Geometry: final body of the model. Coordinates: model frame, mm. A direction names the side the tool comes from. Give positions to 0.01 mm unless a question says otherwise; leave off trailing zeros. Order: outer loops, then holes, each group sorted by start corner. A loop starts at its lowest first (then second) coordinate and runs counter-clockwise, first axis right, second up. Notation, with made-up numbers: M 51,37 L 56,37 A19 ccw 56,60 Z; hole C 66.5,-2 d10. An arc over 180 degrees is marked long. Write item = value, one per line. Start each with the question number.
from build123d import *

# Parameters (mm, degrees)
SKETCH1_R                                     = 19.05
BOSS_EXTRUDE1_DEPTH                           = 2.54
CSK_FOR_4_FLAT_HEAD_MACHINE_SCREW1_AT_2_COUNT = 2
CSK_FOR_4_FLAT_HEAD_MACHINE_SCREW1_AT_2_PITCH = 26.396454307
CSK_FOR_4_FLAT_HEAD_MACHINE_SCREW1_AT_3_COUNT = 2
CSK_FOR_4_FLAT_HEAD_MACHINE_SCREW1_AT_3_PITCH = 26.396454307
F_57_0_043_DIAMETER_HOLE1_D                   = 1.0922
SKETCH9_R                                     = 2.921
BOSS_EXTRUDE2_DEPTH                           = 9.652
CHAMFER1_SIZE                                 = 0.254
F_68_0_031_DIAMETER_HOLE2_D                   = 0.7874
CHAMFER2_SIZE                                 = 0.254
CHAMFER3_SIZE                                 = 0.254
FILLET1_R                                     = 0.381


with BuildPart() as part:
    # Sketch1 → Boss-Extrude1 (new body)
    with BuildSketch(Plane.XY):
        with Locations((-17.766231698, -20.016488826)):
            Circle(SKETCH1_R)
    extrude(amount=BOSS_EXTRUDE1_DEPTH)

    # Sketch2 → CSK for #4 Flat Head Machine Screw1 (revolve, cut)
    with BuildSketch(Plane(origin=(-30.964458851, -27.67786205, 2.54), x_dir=(0, -1, 0), z_dir=(1, 0, 0))):
        Polygon((0, 0), (0, 2.54), (1.63195, 2.54), (1.63195, 1.409834001), (2.8575, 0), align=None)
    csk_for_4_flat_head_machine_screw1 = revolve(axis=Axis((-30.964458851, -27.67786205, 8.89), (0, 0, -1)), mode=Mode.SUBTRACT)

    # CSK for #4 Flat Head Machine Screw1 at 2: CSK for #4 Flat Head Machine Screw1 ×2
    with Locations(*[Vector(0.5, 0.866025404, 0) * (i * CSK_FOR_4_FLAT_HEAD_MACHINE_SCREW1_AT_2_PITCH) for i in range(1, CSK_FOR_4_FLAT_HEAD_MACHINE_SCREW1_AT_2_COUNT)]):
        add(csk_for_4_flat_head_machine_screw1, mode=Mode.SUBTRACT)

    # CSK for #4 Flat Head Machine Screw1 at 3: CSK for #4 Flat Head Machine Screw1 ×2
    with Locations(*[(i * CSK_FOR_4_FLAT_HEAD_MACHINE_SCREW1_AT_3_PITCH, 0, 0) for i in range(1, CSK_FOR_4_FLAT_HEAD_MACHINE_SCREW1_AT_3_COUNT)]):
        add(csk_for_4_flat_head_machine_screw1, mode=Mode.SUBTRACT)

    # #57 (0.043) Diameter Hole1 (through all)
    with Locations(Plane.XY.offset(2.54)):
        with Locations((-17.766231698, -10.81226205), (-25.773156171, -15.43506205), (-9.759307225, -15.43506205), (-8.520631698, -20.05786205), (-9.759307225, -24.68066205), (-17.766231698, -29.30346205), (-25.773156171, -24.68066205)):
            Hole(F_57_0_043_DIAMETER_HOLE1_D / 2)

    # Sketch9 → Boss-Extrude2 (add)
    with BuildSketch(Plane.XY.offset(2.54)):
        with Locations((-12.762431698, -34.829926536)):
            Circle(SKETCH9_R)
    extrude(amount=BOSS_EXTRUDE2_DEPTH)

    # Chamfer1
    chamfer1_edges = [part.edges().sort_by_distance(p)[0] for p in [
        (-25.227056171, -24.68066205, 2.54),
        (-17.220131698, -29.30346205, 2.54),
        (-9.213207225, -24.68066205, 2.54),
        (-7.974531698, -20.05786205, 2.54),
        (-9.213207225, -15.43506205, 2.54),
        (-25.227056171, -15.43506205, 2.54),
        (-17.220131698, -10.81226205, 2.54),
    ]]
    chamfer(chamfer1_edges, length=CHAMFER1_SIZE)

    # #68 (0.031) Diameter Hole2 (through all)
    with Locations(Plane.XY.offset(12.192)):
        with Locations((-13.384731698, -33.752071319), (-13.384731698, -35.907781754), (-11.517831698, -34.829926536)):
            Hole(F_68_0_031_DIAMETER_HOLE2_D / 2)

    # Chamfer2
    chamfer2_edges = [part.edges().sort_by_distance(p)[0] for p in [
        (-11.124131698, -34.829926536, 12.192),
        (-12.991031698, -35.907781754, 12.192),
        (-12.991031698, -33.752071319, 12.192),
    ]]
    chamfer(chamfer2_edges, length=CHAMFER2_SIZE)

    # Chamfer3
    chamfer3_edges = [part.edges().sort_by_distance(p)[0] for p in [
        (-25.227056171, -24.68066205, 0),
        (-17.220131698, -29.30346205, 0),
        (-9.213207225, -24.68066205, 0),
        (-7.974531698, -20.05786205, 0),
        (-9.213207225, -15.43506205, 0),
        (-25.227056171, -15.43506205, 0),
        (-17.220131698, -10.81226205, 0),
        (-11.124131698, -34.829926536, 0),
        (-12.991031698, -35.907781754, 0),
        (-12.991031698, -33.752071319, 0),
    ]]
    chamfer(chamfer3_edges, length=CHAMFER3_SIZE)

    # Fillet1
    fillet1_edges = [part.edges().sort_by_distance(p)[0] for p in [
        (-15.683431698, -34.829926536, 2.54),
    ]]
    fillet(fillet1_edges, radius=FILLET1_R)


solid = part.part
1) Access query for faces 1 (the cylindrical face through (-10.011, -25.165, 1.256)), 2 (the cylindrical face through (-13.4, -37.68, 7.49)). Directions: +Z, -Z, +X, -X, +Y, -Y. A direction counts if a zero-diameter tool reaches every point of the face in a straight line with its end or side. Return the directions, or none.
2) Ray query, L1, parallel to Z at x = -10, y = -23.5; L2, parallel to X at y = -4, z = 0.5; L3, parallel to X at y = -35, z = 8.5. Return the intervals inside material, ascending.
3) Cut plane A-A (z = 4). Return loops of the section in (x, y), plus the area to 3 significant figures.
4) Cut plane C-C (x = -21.5). Return loops of the section in (y, z).
5) Draft query along Y for faces 3 (the cylindrical face through (-36.8, -19.2, 1.3)), 4 (the flat face through (-18, -20, 0)), 5 (the cylindrical face through (-26.025, -15.92, 1.256)), 6 (the cylindrical face through (-10.01, -15.92, 1.26)). Return one class per face: pulls with the +Y half, pulls with the -Y half, needs draft (parallel to the pull), parting line crosses it, or undercut.
6) Pin query (flat end, axial travel): pin 1 Ø1.7 at (x, y) = (-25.77, -15.44) entering from +Z; pin 2 Ø1.3 at (x, y) = (-17.77, -29.3) entering from +Z (3 decimals); pin 3 Ø5 at (x, y) = (-30.96, -27.68) entering from +Z. Return the tip coordinate at first contact, or that it passes through.
7) Cut plane B-B (y = -27.5). Give the number of separate pieces and of enclosed holes in the cut face, plus the area to 3 significant figures.
Reply:
q1.face_1 = +Z, -Z
q1.face_2 = +Z
q2.L1 = 0 to 2.54
q2.L2 = -28.08 to -19.18, -16.35 to -7.45
q2.L3 = -15.68 to -11.87, -11.16 to -9.85
q3.outline = C -12.76,-34.83 d5.84; hole C -13.38,-35.91 d0.79; hole C -13.38,-33.75 d0.79; hole C -11.52,-34.83 d0.79
q3.area = 25.3 mm²
q4.outline = M -38.7,0 L -1.34,0 L -1.34,2.54 L -38.7,2.54 Z
q5.face_3 = parting line crosses it
q5.face_4 = needs draft
q5.face_5 = undercut
q5.face_6 = undercut
q6.pin_1 = 2.54
q6.pin_2 = 2.395
q6.pin_3 = 2.13
q7.separate_pieces = 3
q7.enclosed_holes = 0
q7.area = 69.0 mm²
